from build123d import *

# Parameters (mm, degrees)
SKETCH1_R           = 2.5
SKETCH1_W           = 40
SKETCH1_H           = 40
SKETCH1_R_2         = 1.25
SKETCH1_R_3         = 12.5
BOSS_EXTRUDE1_DEPTH = 2
FILLET1_R           = 50
FILLET2_R           = 20
FILLET3_R           = 8


with BuildPart() as part:
    # Sketch1 → Boss-Extrude1 (new body)
    # profile 1 of 2: a face of its own
    with BuildSketch(Plane(origin=(0, 0, 0), x_dir=(1, 0, 0), z_dir=(0, 1, 0))):
        Polygon((80, 0), (80, 40), (0, 40), (0, 0), (40, 0), align=None)
        with Locations(Location((20, 10, 0), (0, 0, 270))):
            Circle(SKETCH1_R, mode=Mode.SUBTRACT)
        with Locations(Location((20, 30, 0), (0, 0, 270))):
            Circle(SKETCH1_R, mode=Mode.SUBTRACT)
        with Locations(Location((50, 20, 0), (0, 0, 270))):
            Circle(SKETCH1_R, mode=Mode.SUBTRACT)
        with Locations(Location((65, 20, 0), (0, 0, 270))):
            Circle(SKETCH1_R, mode=Mode.SUBTRACT)
    # profile 2 of 2: a face of its own
    with BuildSketch(Plane(origin=(0, 0, 0), x_dir=(1, 0, 0), z_dir=(0, 1, 0))):
        with Locations((20, -20)):
            Rectangle(SKETCH1_W, SKETCH1_H)
        with Locations(Location((4.5, -35.5, 0), (0, 0, 270))):
            Circle(SKETCH1_R_2, mode=Mode.SUBTRACT)
        with Locations(Location((35.5, -35.5, 0), (0, 0, 270))):
            Circle(SKETCH1_R_2, mode=Mode.SUBTRACT)
        with Locations(Location((20, -20, 0), (0, 0, 270))):
            Circle(SKETCH1_R_3, mode=Mode.SUBTRACT)
        with Locations(Location((4.5, -4.5, 0), (0, 0, 270))):
            Circle(SKETCH1_R_2, mode=Mode.SUBTRACT)
        with Locations(Location((35.5, -4.5, 0), (0, 0, 270))):
            Circle(SKETCH1_R_2, mode=Mode.SUBTRACT)
    extrude(amount=BOSS_EXTRUDE1_DEPTH)

    # Fillet1
    # the kernel refuses this fillet: 50 mm, written as the material it adds along each edge
    with BuildSketch(Plane(origin=(40, 0, 0), x_dir=(0, 0, 1), z_dir=(0, 1, 0))) as fillet1_piece_1:
        with BuildLine():
            CenterArc((49.154759474, 49.154759474), FILLET1_R, 190.550098012, 68.899803976)
            Line((0, 40), (0, 0))
            Line((0, 0), (40, 0))
        make_face()
    extrude(amount=2)

    # Fillet2
    fillet2_edges = [part.edges().sort_by_distance(p)[0] for p in [
        (80, 1, -40),
        (80, 1, 0),
        (0, 1, -40),
    ]]
    fillet(fillet2_edges, radius=FILLET2_R)

    # Fillet3
    fillet3_edges = [part.edges().sort_by_distance(p)[0] for p in [
        (40, 1, 40),
        (0, 1, 40),
    ]]
    fillet(fillet3_edges, radius=FILLET3_R)


solid = part.part
Work out the finished part from the listing and answer in its coordinate system (mm). Round coordinates to 2 decimals unless told otherwise and drop trailing zeros. Loops run counter-clockwise (first coordinate to the right, second up) from the corner with the lowest first, then second, coordinate; pieces in that order, holes last. Notation, with made-up numbers: (0, 0.5) - (56, 0.5) arc R31 cw to (56, 25.5) - close; hole circle Ø6 at (24, -13.75). An arc over 180 degrees is marked (long way). Use one line per item in the form item = value. Start each with the question number.
(1) Find section A-A on z = 16. Determine the outline of the cut face in (x, y).
(2) Find section C-C on x = 21.5. Determine the outline of the cut face in (y, z), and give its area (3 significant figures).
(3) Find section D-D on z = 35.5. Determine the outline of the cut face in (x, y).
(4) Flat-ended cylindrical pins translate along their axes: P1, Ø4.5, axis at x = 50, z = -20, coming from the +Y side; P2, Ø1, axis at y = 0.5, z = 22, coming from the +X side. Find the tip coordinate at first contact, or state that the pin passes through.
(5) Find section B-B on y = 1. Give the number of separate pieces and of enclosed holes in the cut face, and give its area (3 significant figures).
(6) Consider line 1 (X direction, y = 1.1, z = -20); line 2 (X direction, y = 1.1, z = 35.5); line 3 (X direction, y = 1.45, z = -8). Determine where each line is inside the solid, lowest interval first.
Answer list:
q1.outline = (0, 0) - (8.16, 0) - (8.16, 2) - (0, 2) - close; (31.84, 0) - (51.73, 0) - (51.73, 2) - (31.84, 2) - close
q2.outline = (0, -40) - (2, -40) - (2, -32) - (0, -32) - close; (0, -28) - (2, -28) - (2, -12) - (0, -12) - close; (0, -8) - (2, -8) - (2, 7.59) - (0, 7.59) - close; (0, 32.41) - (2, 32.41) - (2, 40) - (0, 40) - close
q2.area = 94.4 mm^2
q3.outline = (0.81, 0) - (3.25, 0) - (3.25, 2) - (0.81, 2) - close; (5.75, 0) - (34.25, 0) - (34.25, 2) - (5.75, 2) - close; (36.75, 0) - (40.94, 0) - (40.94, 2) - (36.75, 2) - close
q4.P1 = through
q4.P2 = 47.5
q5.separate_pieces = 1
q5.enclosed_holes = 9
q5.area = 4,450 mm^2
q6.line_1 = 0 to 47.5, 52.5 to 62.5, 67.5 to 80
q6.line_2 = 0.81 to 3.25, 5.75 to 34.25, 36.75 to 40.94
q6.line_3 = 0 to 18.5, 21.5 to 78.92
